Verification items for this drawing (mm, ordinates from the low corner). A direction names the side the tool comes from. Round coordinates to 2 decimals unless told otherwise and drop trailing zeros. Loops run counter-clockwise (first coordinate to the right, second up) from the corner with the lowest first, then second, coordinate; pieces in that order, holes last. Notation, with made-up numbers: (-35, 13) -> (-29, 13) arc R35 cw to (-29, 48) -> close; hole circle Ø9 at (-24, -34). An arc over 180 degrees is marked (long way). Use a Markdown table: item, result. Add a question column.
Q1. Sectioned sample at A-A, the plane z = 2.9. Enter the section's corners in (x, y).
Q2. Set-up check for the marked faces 1 and 2: record each of +Z, -Z, +X, -X, +Y, -Y from which the full face is reachable in a straight line by a thin tool's end or side.
Q3. Release check for a two-part mould opening along Y. For the marked faces 3, 4 and 5 record: released by +Y, released by -Y, zero draft, split by the parting line, or undercut.
Q4. Material ranges on L1, parallel to X at y = 2, z = 3.35 (1 decimal); L2, parallel to X at y = 4.05, z = 1.75 (1 decimal); L3, parallel to Y at x = 3.4, z = 2.4 (1 decimal), recorded low to high.
Q5. Gauge pin test, flat ends, axial feed: P1, Ø2, axis at x = 2.73, y = 2.98, coming from the -Z side; P2, Ø1.5, axis at y = 3.5, z = 2, coming from the +X side. Record the tip position at first contact, or that the pin passes through.
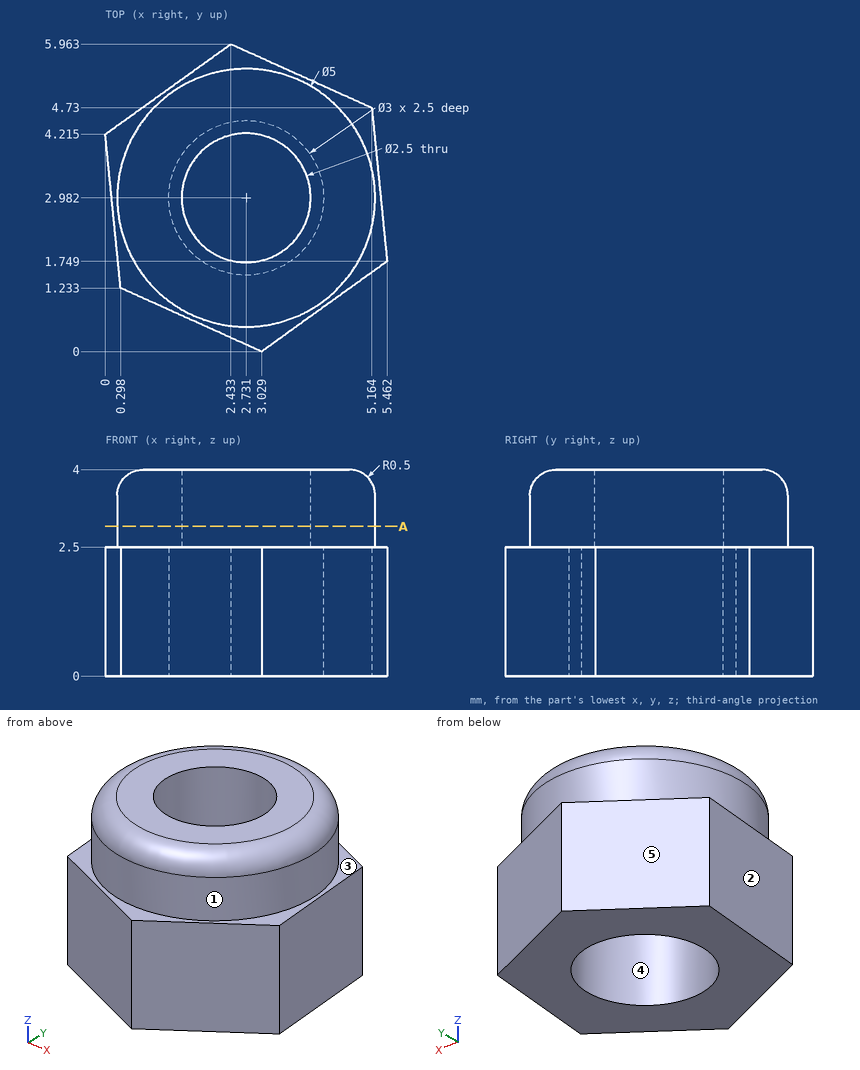
Values:
| question | item | result |
|---|---|---|
| 1 | outline | circle Ø5 at (2.73, 2.98); hole circle Ø2.5 at (2.73, 2.98) |
| 2 | face 1 | +Z |
| 2 | face 2 | +Z, -Z, -X, -Y |
| 3 | face 3 | zero draft |
| 3 | face 4 | undercut |
| 3 | face 5 | released by +Y |
| 4 | L1 | 0.4 to 2, 3.5 to 5 |
| 4 | L2 | 0 to 1.7, 3.8 to 5.2 |
| 4 | L3 | 0.3 to 1.6, 4.3 to 5.5 |
| 5 | P1 | through |
| 5 | P2 | x = 5.36 |
